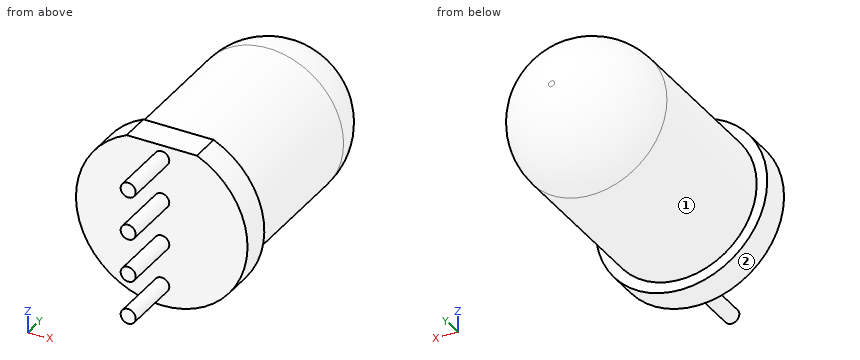
```python
from build123d import *

# Parameters (mm, degrees)
CUT_EXTRUDE1_DEPTH  = 1
SKETCH3_R           = 0.25
BOSS_EXTRUDE1_DEPTH = 2


with BuildPart() as part:
    # Sketch1 → Revolve1 (revolve)
    with BuildSketch(Plane.XY):
        with BuildLine():
            Line((0, 0), (0, 8.75))
            Line((0, 8.75), (0.1, 8.75))
            ThreePointArc((0.1, 8.75), (1.797056275, 8.047056275), (2.5, 6.35))
            Line((2.5, 6.35), (2.5, 1))
            Line((2.5, 1), (2.85, 1))
            Line((2.85, 1), (2.85, 0))
            Line((2.85, 0), (0, 0))
        make_face()
    revolve(axis=Axis((0, 0, 0), (0, 1, 0)))

    # Sketch2 → Cut-Extrude1 (cut)
    with BuildSketch(Plane.XZ):
        with BuildLine():
            Line((-1.167261753, 2.6), (1.167261753, 2.6))
            ThreePointArc((1.167261753, 2.6), (0, 2.85), (-1.167261753, 2.6))
        make_face()
    extrude(amount=-CUT_EXTRUDE1_DEPTH, mode=Mode.SUBTRACT)

    # Sketch3 → Boss-Extrude1 (add)
    with BuildSketch(Plane.XZ):
        with Locations((0, -2.15)):
            Circle(SKETCH3_R)
        with Locations((0, 2.15)):
            Circle(SKETCH3_R)
        with Locations((0, -0.716666667)):
            Circle(SKETCH3_R)
        with Locations((0, 0.716666667)):
            Circle(SKETCH3_R)
    extrude(amount=BOSS_EXTRUDE1_DEPTH)


solid = part.part
```
Verification items for the finished model (mm, model axes). Face numbers are marked on the shaded views. A direction names the side the tool comes from. Round coordinates to 2 decimals unless told otherwise and drop trailing zeros. Write each loop counter-clockwise with the first axis right and the second up, starting at its lowest first coordinate (ties: lowest second). Pieces come first, ordered by that corner, then holes. Notation, with made-up numbers: (68, 57.25) - (114, 57.25) arc R16 cw to (114, 80.25) - close; hole circle Ø8 at (-9.75, -25). An arc over 180 degrees is marked (long way). Answer as a JSON object with one key per item and string values. Group by question number.
Q1. Section check A-A, the plane y = -0.75. Enter the section's corners in (x, z), plus the area to 3 significant figures.
Q2. Go/stop test with flat-tipped pins: pin 1 Ø1 at (x, z) = (1.5, -1) entering from -Y; pin 2 Ø1.5 at (x, y) = (2, 2) entering from +Z; pin 3 Ø1 at (x, y) = (-0.5, 6) entering from -Z. Record where each tip stops, or that it passes through.
Q3. Tool access check on the marked faces 1 and 2. Record the directions out of +Z, -Z, +X, -X, +Y, -Y that give a thin tool (end or side, any length) a straight path to the whole face; none if there is none.
Q4. Thickness scan on line 1 (Y direction, x = -2.3, z = -1.5); line 2 (Y direction, x = 0.4, z = 0.45); line 3 (Z direction, x = 0.7, y = 2). Record the ranges inside material, lowest first.
Found:
{
 "1": {"outline": "circle Ø0.5 at (0, -2.15); circle Ø0.5 at (0, -0.72); circle Ø0.5 at (0, 0.72); circle Ø0.5 at (0, 2.15)", "area": "0.785 mm^2"},
 "2": {"pin 1": "stops at y = 0", "pin 2": "stops at z = 2.17", "pin 3": "stops at z = -2.5"},
 "3": {"face 1": "+Y", "face 2": "+Y, -Y"},
 "4": {"line 1": "y = 0 to 1", "line 2": "y = 0 to 8.7", "line 3": "z = -2.4 to 2.4"}
}
